Part model, mm, in its own coordinate system. Face numbers are marked on the shaded views. A direction names the side the tool comes from. Give positions to 0.01 mm unless a question says otherwise; leave off trailing zeros. Order: outer loops, then holes, each group sorted by start corner. A loop starts at its lowest first (then second) coordinate and runs counter-clockwise, first axis right, second up. Notation, with made-up numbers: M 63,-24 L 107,-24 A12 cw 107,-8 Z; hole C 52,-5 d9. An arc over 180 degrees is marked long. Return JSON: item names as keys, results as strings.
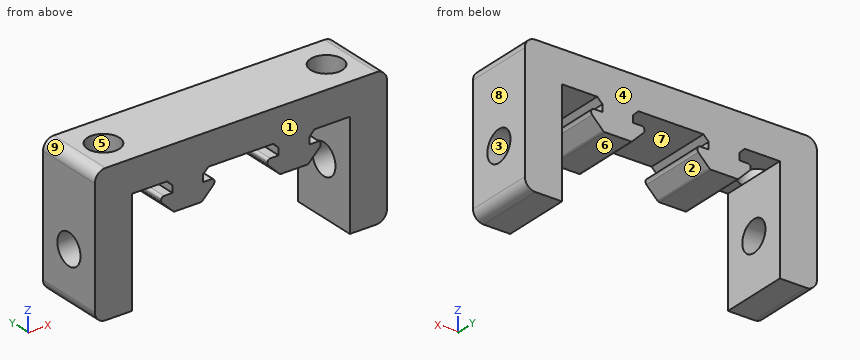
from build123d import *

# Parameters (mm, degrees)
SKETCH1_W            = 55
SKETCH1_H            = 13
BOSS_EXTRUDE1_DEPTH  = 10
SKETCH2_W            = 55
SKETCH2_H            = 13
CUT_EXTRUDE1_DEPTH   = 4
CUT_EXTRUDE2_REACH   = 30.888
SKETCH4_R            = 3
BOSS_EXTRUDE3_DEPTH  = 13
SKETCH6_W            = 7
SKETCH6_H            = 13
BOSS_EXTRUDE4_DEPTH  = 20
M5_CLEARANCE_HOLE1_D = 5.8
FILLET1_R            = 2
FILLET2_R            = 0.5


with BuildPart() as part:
    # Sketch1 → Boss-Extrude1 (new body)
    with BuildSketch(Plane.XY):
        Rectangle(SKETCH1_W, SKETCH1_H)
    extrude(amount=BOSS_EXTRUDE1_DEPTH)

    # Sketch2 → Cut-Extrude1 (cut)
    with BuildSketch(Plane.XY.offset(10)):
        Rectangle(SKETCH2_W, SKETCH2_H)
    extrude(amount=-CUT_EXTRUDE1_DEPTH, mode=Mode.SUBTRACT)

    # Sketch4 → Cut-Extrude2 (cut, up to next)
    with BuildSketch(Plane.XY.offset(6), mode=Mode.PRIVATE) as cut_extrude2_sk1:
        with Locations((21, 0)):
            Circle(SKETCH4_R)
    cut_extrude2_tool1 = extrude(cut_extrude2_sk1.sketch, amount=-CUT_EXTRUDE2_REACH, mode=Mode.PRIVATE) & part.part
    # Sketch4 → Cut-Extrude2 (cut, up to next)
    with BuildSketch(Plane.XY.offset(6), mode=Mode.PRIVATE) as cut_extrude2_sk2:
        with Locations((-21, 0)):
            Circle(SKETCH4_R)
    cut_extrude2_tool2 = extrude(cut_extrude2_sk2.sketch, amount=-CUT_EXTRUDE2_REACH, mode=Mode.PRIVATE) & part.part
    add(cut_extrude2_tool1.solids().sort_by_distance((21, 0, 6))[0], mode=Mode.SUBTRACT)
    add(cut_extrude2_tool2.solids().sort_by_distance((-21, 0, 6))[0], mode=Mode.SUBTRACT)

    # Sketch5 → Boss-Extrude3 (add)
    with BuildSketch(Plane(origin=(0, 6.5, 0), x_dir=(1, 0, 0), z_dir=(0, 1, 0))):
        Polygon((9.9, 5.5995), (12.632393219, 5.5995), (15, 3.231893219), (15, 2.3), (12.8865, 2.3), (12.8865, 0.982893219), (13.869393219, 0), (6.130606781, 0), (7.1135, 0.982893219), (7.1135, 2.3), (5, 2.3), (5, 3.231893219), (7.367606781, 5.5995), align=None)
    boss_extrude3 = extrude(amount=-BOSS_EXTRUDE3_DEPTH)

    # Mirror1: Boss-Extrude3 across plane
    add(boss_extrude3.mirror(Plane(origin=(0, 0, 0), x_dir=(0, 0, 1), z_dir=(1, 0, 0))))

    # Sketch6 → Boss-Extrude4 (add)
    with BuildSketch(Plane(origin=(0, 0, 0), x_dir=(-1, 0, 0), z_dir=(0, 0, -1))):
        with Locations((24, 0)):
            Rectangle(SKETCH6_W, SKETCH6_H)
        with Locations((-24, 0)):
            Rectangle(SKETCH6_W, SKETCH6_H)
    extrude(amount=BOSS_EXTRUDE4_DEPTH)

    # M5 Clearance Hole1 (through all)
    with Locations(Plane(origin=(-27.5, 0, -10), x_dir=(0, 0, -1), z_dir=(-1, 0, 0))):
        with Locations((0, 0)):
            Hole(M5_CLEARANCE_HOLE1_D / 2)

    # Fillet1
    fillet1_edges = [part.edges().sort_by_distance(p)[0] for p in [
        (-27.5, 0, -20),
        (27.5, 0, -20),
        (-27.5, 0, 6),
        (27.5, 0, 6),
    ]]
    fillet(fillet1_edges, radius=FILLET1_R)

    # Fillet2
    fillet2_edges = [part.edges().sort_by_distance(p)[0] for p in [
        (12.632393219, 0, -5.5995),
        (15, 0, -3.231893219),
        (15, 0, -2.3),
        (5, 0, -2.3),
        (5, 0, -3.231893219),
        (7.367606781, 0, -5.5995),
        (-15, 0, -2.3),
        (-5, 0, -2.3),
        (-5, 0, -3.231893219),
        (-7.367606781, 0, -5.5995),
        (-12.632393219, 0, -5.5995),
        (-15, 0, -3.231893219),
    ]]
    fillet(fillet2_edges, radius=FILLET2_R)


solid = part.part
Q1. Band-saw the part on C-C (x = 20). Give the cut face in (y, z).
Established:
{"outline": "M -6.5,0 L -2.83,0 L -2.83,6 L -6.5,6 Z; M 2.83,0 L 6.5,0 L 6.5,6 L 2.83,6 Z"}
Q2. 3-axis set-ups, long thin cutter, end or side, ignore diameter. For the marked faces 5, 6, 7, 8 and 9: which of +Z, -Z, +X, -X, +Y, -Y reach the whole face in a straight line?
Established:
{"face 5": "+Z", "face 6": "-Z, +Y, -Y", "face 7": "+Y, -Y", "face 8": "+Z, -Z, +X, +Y, -Y", "face 9": "+Z, -X, +Y, -Y"}
Q3. Band-saw the part on B-B (x = -23). Give the cut face in (y, z), then the cut area to 3 significant figures.
Established:
{"outline": "M -6.5,-20 L 6.5,-20 L 6.5,6 L 2.24,6 L 2.24,0 L -2.24,0 L -2.24,6 L -6.5,6 Z; hole C 0,-10 d5.8", "area": "285 mm²"}
Q4. Two-plate mould, pull along Y, no slides. Class the marked faces 1, 2, 3 and 4: +Y half, -Y half, draft (parallel to the pull), parting line (faces both ways), or undercut.
Established:
{"face 1": "-Y half", "face 2": "draft", "face 3": "undercut", "face 4": "+Y half"}
Q5. Probe line 1 along X through (y, z) = (5.75, -15.25); line 2 along X through (y, z) = (-3.25, -4); line 3 along X through (y, z) = (-5, -0.5). List the from-to ranges inside material, lowest first.
Established:
{"line 1": "x = -27.5 to -20.5, 20.5 to 27.5", "line 2": "x = -27.5 to -20.5, -14.23 to -5.77, 5.77 to 14.23, 20.5 to 27.5", "line 3": "x = -27.5 to -20.5, -13.37 to -6.63, 6.63 to 13.37, 20.5 to 27.5"}
Q6. Pin check, flat tips, straight feed: pin 1 (3.5 mm diameter, centred on x = 18.5, y = 2.5, fed in from -Z); pin 2 (5.5 mm diameter, centred on x = 10.5, y = -1, fed in from -Z). Stop position of each tip, or through.
Established:
{"pin 1": "stops at z = 0", "pin 2": "stops at z = -5.6"}
Q7. Band-saw the part on D-D (y = 0). Give the number of separate pieces and of enclosed holes in the cut face, then the cut area to 3 significant figures.
Established:
{"separate pieces": "5", "enclosed holes": "0", "area": "536 mm²"}
Q8. Band-saw the part on A-A (z = -10). Give the cut face in (x, y), then the cut area to 3 significant figures.
Established:
{"outline": "M -27.5,-6.5 L -20.5,-6.5 L -20.5,-2.9 L -27.5,-2.9 Z; M -27.5,2.9 L -20.5,2.9 L -20.5,6.5 L -27.5,6.5 Z; M 20.5,-6.5 L 27.5,-6.5 L 27.5,-2.9 L 20.5,-2.9 Z; M 20.5,2.9 L 27.5,2.9 L 27.5,6.5 L 20.5,6.5 Z", "area": "101 mm²"}
